from build123d import *

# Parameters (mm, degrees)
F0_W     = 265
F0_H     = 50
F1_DEPTH = 15
F2_W     = 20
F2_H     = 40
F3_DEPTH = 39.9
F4_DEPTH = 35.1


with BuildPart() as f1:
    # F0 (on Top) → F1 (new body)
    with BuildSketch(Plane.XY):
        with Locations((0, 1.633065)):
            Rectangle(F0_W, F0_H)
    extrude(amount=F1_DEPTH)

    # F2 (on face) → F3 (cut)
    with BuildSketch(Plane.XY.offset(15)):
        with Locations((-62.5, 1.633065)):
            Rectangle(F2_W, F2_H)
        with Locations((62.5, 1.633065)):
            Rectangle(F2_W, F2_H)
    extrude(amount=-F3_DEPTH, mode=Mode.SUBTRACT)

    # F2 (on face) → F4 (cut)
    with BuildSketch(Plane.XY.offset(15)):
        with Locations((-62.5, 1.633065)):
            Rectangle(F2_W, F2_H)
        with Locations((62.5, 1.633065)):
            Rectangle(F2_W, F2_H)
    extrude(amount=-F4_DEPTH, mode=Mode.SUBTRACT)


solid = f1.part
Verification items for the finished model (mm, model axes). A direction names the side the tool comes from. Round coordinates to 2 decimals unless told otherwise and drop trailing zeros. Loops run counter-clockwise (first coordinate to the right, second up) from the corner with the lowest first, then second, coordinate; pieces in that order, holes last. Notation, with made-up numbers: (61.25, -27) - (85.25, -27) arc R7 ccw to (85.25, -14) - close; hole circle Ø7 at (56, -15). An arc over 180 degrees is marked (long way). Use one line per item in the form item = value.
1. Scan lines: probe 1 along X at (y, z) = (-13.5, 7.5); probe 2 along Y at (x, z) = (56, 8.5). Record each from-to range of solid material in increasing order.
A:
probe_1 = -132.5 to -72.5, -52.5 to 52.5, 72.5 to 132.5
probe_2 = -23.37 to -18.37, 21.63 to 26.63
2. Section check A-A on y = 14.5. Record the cut outline in (x, z).
A:
outline = (-132.5, 0) - (-72.5, 0) - (-72.5, 15) - (-132.5, 15) - close; (-52.5, 0) - (52.5, 0) - (52.5, 15) - (-52.5, 15) - close; (72.5, 0) - (132.5, 0) - (132.5, 15) - (72.5, 15) - close
3. Gauge pin test, flat end, axial feed: pin 1 Ø4 at (x, y) = (-58.5, 18.5) entering from -Z. Record the tip position at first contact, or that the pin passes through.
A:
pin_1 = through
4. Draft check along X on faces 3 (the flat face through (-72.5, 1, 8)), 4 (the flat face through (132.5, 1, 7)), 5 (the flat face through (-132.5, 1, 7)). Enter one of: pulls with the +X half, pulls with the -X half, needs draft (parallel to the pull), parting line crosses it, or undercut.
A:
face_3 = undercut
face_4 = pulls with the +X half
face_5 = pulls with the -X half
5. Section check B-B on z = 6.75. Record the cut outline in (x, y), and give its area (4 significant figures).
A:
outline = (-132.5, -23.37) - (132.5, -23.37) - (132.5, 26.63) - (-132.5, 26.63) - close; hole (-72.5, -18.37) - (-52.5, -18.37) - (-52.5, 21.63) - (-72.5, 21.63) - close; hole (52.5, -18.37) - (72.5, -18.37) - (72.5, 21.63) - (52.5, 21.63) - close
area = 11,650 mm²
6. Access from +Z, -Z, +X, -X, +Y, -Y to the whole of each face (thin tool, end or side, straight path). Record for faces 1 (the flat face through (-2, 2, 15)), 2 (the flat face through (62, 21.633, 8)).
A:
face_1 = +Z, +X, -X, +Y, -Y
face_2 = +Z, -Z
